from build123d import *

# Parameters (mm, degrees)
SKETCH1_R           = 57.5
BOSS_EXTRUDE1_DEPTH = 4
BOSS_EXTRUDE2_DEPTH = 4
CUT_EXTRUDE1_DEPTH  = 5
CUT_EXTRUDE2_DEPTH  = 5
SKETCH5_R           = 43.5
CUT_EXTRUDE3_DEPTH  = 5
CUT_EXTRUDE7_DEPTH  = 5
SKETCH9_R           = 1.25
CUT_EXTRUDE10_DEPTH = 5
CUT_EXTRUDE14_DEPTH = 5


with BuildPart() as part:
    # Sketch1 → Boss-Extrude1 (new body)
    with BuildSketch(Plane(origin=(0, 0, 0), x_dir=(1, 0, 0), z_dir=(0, 1, 0))):
        Circle(SKETCH1_R)
    extrude(amount=BOSS_EXTRUDE1_DEPTH)

    # Sketch2 → Boss-Extrude2 (add)
    with BuildSketch(Plane(origin=(0, 0, 0), x_dir=(1, 0, 0), z_dir=(0, 1, 0))):
        Polygon((-77.977903645, -19.095954082), (-57.5, 0), (-44.924411203, 0), (-44.924411203, 25.803568088), (-64.346784729, 10.023199482), (-86.161883966, -10.319709662), align=None)
    extrude(amount=BOSS_EXTRUDE2_DEPTH)

    # Sketch3 → Cut-Extrude1 (cut, through all)
    with BuildSketch(Plane(origin=(0, 0, 0), x_dir=(1, 0, 0), z_dir=(0, 1, 0))):
        with BuildLine():
            ThreePointArc((-51.43555025, 13.782114152), (-35.975178556, 39.260018185), (-9.246765461, 52.441012848))
            ThreePointArc((-9.246765461, 52.441012848), (-6.640239617, 50.615903803), (-8.465348661, 48.009377959))
            ThreePointArc((-8.465348661, 48.009377959), (-32.935022621, 35.942270169), (-47.088884032, 12.617428449))
            ThreePointArc((-47.088884032, 12.617428449), (-49.844559992, 11.026438191), (-51.43555025, 13.782114152))
        make_face()
    extrude(amount=CUT_EXTRUDE1_DEPTH, mode=Mode.SUBTRACT)

    # Sketch4 → Cut-Extrude2 (cut, through all)
    with BuildSketch(Plane(origin=(0, 0, 0), x_dir=(1, 0, 0), z_dir=(0, 1, 0))):
        with BuildLine():
            Line((0, 0), (-57.5, 0))
            ThreePointArc((-57.5, 0), (42.393446867, -38.846436938), (-5.011455208, 57.28119514))
            Line((-5.011455208, 57.28119514), (0, 0))
        make_face()
    extrude(amount=CUT_EXTRUDE2_DEPTH, mode=Mode.SUBTRACT)

    # Sketch5 → Cut-Extrude3 (cut, through all)
    with BuildSketch(Plane(origin=(0, 0, 0), x_dir=(1, 0, 0), z_dir=(0, 1, 0))):
        Circle(SKETCH5_R)
    extrude(amount=CUT_EXTRUDE3_DEPTH, mode=Mode.SUBTRACT)

    # Sketch7 → Cut-Extrude7 (cut, through all)
    with BuildSketch(Plane(origin=(0, 0, 0), x_dir=(1, 0, 0), z_dir=(0, 1, 0))):
        Polygon((-57.5, 0), (-41.603937585, 12.702849184), (-43.5, 0), align=None)
    extrude(amount=CUT_EXTRUDE7_DEPTH, mode=Mode.SUBTRACT)

    # Sketch9 → Cut-Extrude10 (cut, through all)
    with BuildSketch(Plane(origin=(0, 4, 0), x_dir=(1, 0, 0), z_dir=(0, 1, 0))):
        with Locations((-76.485000828, -14.098640015)):
            Circle(SKETCH9_R)
        with Locations((-71.66338638, -5.91316299)):
            Circle(SKETCH9_R)
    extrude(amount=-CUT_EXTRUDE10_DEPTH, mode=Mode.SUBTRACT)

    # Sketch10 → Cut-Extrude14 (cut, through all)
    with BuildSketch(Plane(origin=(0, 4, 0), x_dir=(1, 0, 0), z_dir=(0, 1, 0))):
        with BuildLine():
            ThreePointArc((-75.78838638, -13.057872572), (-77.983253036, -11.21616077), (-79.415850502, -8.734829173))
            ThreePointArc((-79.415850502, -8.734829173), (-81.017991457, -7.987738576), (-81.765082054, -9.589879531))
            ThreePointArc((-81.765082054, -9.589879531), (-79.898364144, -12.823129794), (-77.03838638, -15.222936081))
            ThreePointArc((-77.03838638, -15.222936081), (-75.330854625, -14.765404326), (-75.78838638, -13.057872572))
        make_face()
    extrude(amount=-CUT_EXTRUDE14_DEPTH, mode=Mode.SUBTRACT)


solid = part.part
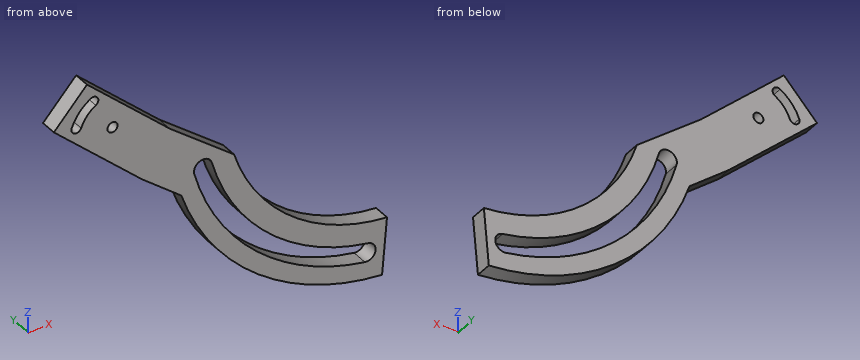
Work out the finished part from the listing and answer in its coordinate system (mm). Give positions to 0.01 mm unless a question says otherwise; leave off trailing zeros. Loops run counter-clockwise (first coordinate to the right, second up) from the corner with the lowest first, then second, coordinate; pieces in that order, holes last. Notation, with made-up numbers: (-34.75, 34.25) - (14.25, 34.25) arc R11 cw to (14.25, 48.25) - close; hole circle Ø6 at (78.25, -11). An arc over 180 degrees is marked (long way). Answer in a Markdown table with one row per item.
(1) Section B-B (x = -45) is taken. Give the vertices of the cut face in (y, z).
Results list:
| item | result |
|---|---|
| outline | (0, -35.79) - (4, -35.79) - (4, -28.47) - (0, -28.47) - close; (0, -18.75) - (4, -18.75) - (4, -9.99) - (0, -9.99) - close |
(2) Section D-D (z = 3.5) is taken. Give the vertices of the cut face in (x, y), and give its area (3 significant figures).
Results list:
| item | result |
|---|---|
| outline | (-78.85, 0) - (-61.25, 0) - (-61.25, 4) - (-78.85, 4) - close |
| area | 70.4 mm² |
(3) Section C-C (y = 2.3) is taken. Give the vertices of the cut face in (x, z).
Results list:
| item | result |
|---|---|
| outline | (-86.16, 10.32) - (-64.35, -10.02) - (-54.64, -17.91) arc R57.5 ccw to (-5.01, -57.28) - (-3.79, -43.33) arc R43.5 cw to (-41.6, -12.7) - (-57.5, 0) - (-77.98, 19.1) - close; hole (-81.77, 9.59) arc R1.25 ccw to (-79.42, 8.73) arc R8.25 cw to (-75.79, 13.06) arc R1.25 ccw to (-77.04, 15.22) arc R10.75 ccw to start; hole circle Ø2.5 at (-71.66, 5.91); hole (-51.44, -13.78) arc R53.25 ccw to (-9.25, -52.44) arc R2.25 ccw to (-8.47, -48.01) arc R48.75 cw to (-47.09, -12.62) arc R2.25 ccw to start |
(4) Flat-ended cylindrical pins translate along their axes: pin 1 Ø2 at (x, y) = (-53.5, 0.5) entering from -Z; pin 2 Ø1 at (y, z) = (3.5, 3.5) entering from -X; pin 3 Ø2 at (x, z) = (-71.66, 5.91) entering from +Y. Find the tip coordinate at first contact, or state that the pin passes through.
Results list:
| item | result |
|---|---|
| pin 1 | stops at z = -23.45 |
| pin 2 | stops at x = -79.38 |
| pin 3 | passes through |
(5) Section A-A (z = -50) is taken. Give the vertices of the cut face in (x, y), and give its area (3 significant figures).
Results list:
| item | result |
|---|---|
| outline | (-28.39, 0) - (-18.32, 0) - (-18.32, 4) - (-28.39, 4) - close; (-6.62, 0) - (-4.37, 0) - (-4.37, 4) - (-6.62, 4) - close |
| area | 49.3 mm² |
(6) Consider L1, parallel to X at y = 0.7, z = -22; L2, parallel to X at y = 2.15, z = -14; L3, parallel to Z at x = -32, y = 3.4. Determine where each line is inside the solid, lowest interval first. Write a range as [from, to].
Results list:
| item | result |
|---|---|
| L1 | x = [-53.12, -48.49], [-43.5, -37.53] |
| L2 | x = [-59.45, -51.38], [-46.7, -41.19] |
| L3 | z = [-47.77, -42.56], [-36.78, -29.47] |
